from build123d import *

# Parameters (mm, degrees)
PAD006_DEPTH      = 10
CYLINDER010_R     = 5
CYLINDER010_DEPTH = 15
PAD_DEPTH         = 6.5
PAD001_DEPTH      = 4
PAD002_DEPTH      = 10
CYLINDER011_R     = 8
CYLINDER011_DEPTH = 5


with BuildPart() as body004:
    # Sketch006 → Pad006 (new body)
    with BuildSketch(Plane.XY):
        Polygon((0, -2.5), (-1, -2.5), (-1, -1), (-2.5, -1), (-2.5, 0), (-2.5, 1), (-1, 1), (-1, 2.5), (0, 2.5), (1, 2.5), (1, 1), (2.5, 1), (2.5, 0), (2.5, -1), (1, -1), (1, -2.5), align=None)
    extrude(amount=PAD006_DEPTH)


with BuildPart() as body004_1:
    # Body004 placement: moved
    add(body004.part.moved(Location((0, 0, 15))))


with BuildPart() as cut010:
    # Cylinder010 → Cylinder010 (new body)
    with BuildSketch(Plane.XY.offset(10)):
        Circle(CYLINDER010_R)
    extrude(amount=CYLINDER010_DEPTH)

    # Cut010: cut Body004
    add(body004_1.part, mode=Mode.SUBTRACT)


with BuildPart() as cuerpo:
    # Sketch → Pad (new body)
    with BuildSketch(Plane.XY):
        Polygon((0, 7.505553), (-6.5, 3.752777), (-6.5, -3.752777), (0, -7.505553), (6.5, -3.752777), (6.5, 3.752777), align=None)
    extrude(amount=PAD_DEPTH)

    # Sketch001 (on Face8 of Pad) → Pad001 (join)
    with BuildSketch(Plane.XY.offset(6.5)):
        Polygon((0, 5.773503), (-5, 2.886751), (-5, -2.886751), (0, -5.773503), (5, -2.886751), (5, 2.886751), align=None)
    extrude(amount=PAD001_DEPTH)


with BuildPart() as cut009:
    # Sketch002 → Pad002 (new body)
    with BuildSketch(Plane.XY):
        Polygon((0, 9.814955), (-8.5, 4.907477), (-8.5, -4.907477), (0, -9.814955), (8.5, -4.907477), (8.5, 4.907477), align=None)
    extrude(amount=PAD002_DEPTH)

    # Cut009: cut Cuerpo
    add(cuerpo.part, mode=Mode.SUBTRACT)


with BuildPart() as union_motor:
    # Cylinder011 → Cylinder011 (new body)
    with BuildSketch(Plane.XY.offset(10)):
        Circle(CYLINDER011_R)
    extrude(amount=CYLINDER011_DEPTH)

    # Fusion004: union Cut010, Cut009
    add(cut010.part)
    add(cut009.part)


solid = union_motor.part
Work out the finished part from the listing and answer in its coordinate system (mm). A direction names the side the tool comes from. Give positions to 0.01 mm unless a question says otherwise; leave off trailing zeros. Write each loop counter-clockwise with the first axis right and the second up, starting at its lowest first coordinate (ties: lowest second). Pieces come first, ordered by that corner, then holes.
Q1. The part is cut by section B-B on x = 6. Give the vertices of the cut face in (y, z).
Answer:
outline: (-6.35, 0) - (-4.04, 0) - (-4.04, 6.5) - (4.04, 6.5) - (4.04, 0) - (6.35, 0) - (6.35, 10) - (5.29, 10) - (5.29, 15) - (-5.29, 15) - (-5.29, 10) - (-6.35, 10) - close
Q2. Given pin 1 (1.2 mm diameter, centred on x = -1.5, z = 21.5, fed in from -Y); pin 2 (8 mm diameter, centred on y = -1, z = 17.5, fed in from -X); pin 3 (1.2 mm diameter, centred on y = 2, z = 22, fed in from +X), each flat-ended and moving along its own axis, determine where each tip first touches the part or whether it passes through.
Answer:
pin 1: stops at y = -4.92
pin 2: stops at x = -8
pin 3: stops at x = 4.8
Q3. A tool of negligible diameter and unlimited length cuts with its end or side. For faces 1 (the face through (0, 0, 10)), 2 (the face through (4.19, -7.396, 4.93)), 3 (the face through (2, -1, 20)), from which of +Z, -Z, +X, -X, +Y, -Y can it reach the whole face along a straight path? Write none if from no direction.
Answer:
face 1: -Z
face 2: +Z, -Z, +X, -Y
face 3: +Z
Q4. The part is cut by section D-D on x = 3. Give the vertices of the cut face in (y, z), and give its area (3 significant figures).
Answer:
outline: (-8.08, 0) - (-5.77, 0) - (-5.77, 6.5) - (-4.04, 6.5) - (-4.04, 10) - (4.04, 10) - (4.04, 6.5) - (5.77, 6.5) - (5.77, 0) - (8.08, 0) - (8.08, 10) - (7.42, 10) - (7.42, 15) - (4, 15) - (4, 25) - (-4, 25) - (-4, 15) - (-7.42, 15) - (-7.42, 10) - (-8.08, 10) - close
area: 212 mm2
Q5. Straight lines are drawn through the part: L1, parallel to X at y = 0, z = 19.75; L2, parallel to X at y = 2, z = 3; L3, parallel to Z at x = 8.25, y = -4.25. For each, find the intervals that lie inside material, in ascending order.
Answer:
L1: x = -5 to -2.5, 2.5 to 5
L2: x = -8.5 to -6.5, 6.5 to 8.5
L3: z = 0 to 10
Q6. The part is cut by section C-C on z = 14.25. Give the vertices of the cut face in (x, y).
Answer:
outline: circle Ø16 at (0, 0)
Q7. For a pull along X with two mould halves and no side action, classify faces 4 (the face through (-4.31, -7.327, 4.93)), 5 (the face through (8.5, 0, 5)), 6 (the face through (2, 1, 20)) as released by +X, released by -X, zero draft, split by the parting line, or undercut.
Answer:
face 4: released by -X
face 5: released by +X
face 6: undercut
Q8. The part is cut by section A-A on y = 0. Give the vertices of the cut face in (x, z).
Answer:
outline: (-8.5, 0) - (-6.5, 0) - (-6.5, 6.5) - (-5, 6.5) - (-5, 10) - (5, 10) - (5, 6.5) - (6.5, 6.5) - (6.5, 0) - (8.5, 0) - (8.5, 10) - (8, 10) - (8, 15) - (5, 15) - (5, 25) - (2.5, 25) - (2.5, 15) - (-2.5, 15) - (-2.5, 25) - (-5, 25) - (-5, 15) - (-8, 15) - (-8, 10) - (-8.5, 10) - close
